```python
from build123d import *

# Parameters (mm, degrees)
SKETCH_1_W           = 10
SKETCH_1_H           = 10
EXTRUDE_2_DEPTH      = 10
EXTRUDE_2_2_DEPTH    = 10
EXTRUDE_2_3_DEPTH    = 10
EXTRUDE_2_4_DEPTH    = 10
SKETCH_2_W           = 100
SKETCH_2_H           = 50
EXTRUDE_3_DEPTH      = 5
SKETCH_4_W           = 100
SKETCH_4_H           = 5
EXTRUDE_4_DEPTH      = 50
SKETCH_7_R           = 4
CUT_EXTRUDE_7_DEPTH  = 100
SKETCH_8_W           = 84
SKETCH_8_H           = 34
CUT_EXTRUDE_9_DEPTH  = 5
CUT_EXTRUDE_12_REACH = 78.195
SKETCH_10_W          = 7
SKETCH_10_H          = 2
CUT_EXTRUDE_13_REACH = 78.195
SKETCH_12_W          = 7
SKETCH_12_H          = 2


with BuildPart() as part:
    # Sketch 1 → Extrude 2 (new body)
    with BuildSketch(Plane(origin=(0, 0, 0), x_dir=(1, 0, 0), z_dir=(0, 1, 0))):
        with Locations((-31.40167364, 31.889818689)):
            Rectangle(SKETCH_1_W, SKETCH_1_H)
    extrude(amount=EXTRUDE_2_DEPTH)



with BuildPart() as body_2:
    # Sketch 1 → Extrude 2 2 (new body)
    with BuildSketch(Plane(origin=(0, 0, 0), x_dir=(1, 0, 0), z_dir=(0, 1, 0))):
        with Locations((-31.40167364, -8.110181311)):
            Rectangle(SKETCH_1_W, SKETCH_1_H)
    extrude(amount=EXTRUDE_2_2_DEPTH)


with BuildPart() as body_3:
    # Sketch 1 → Extrude 2 3 (new body)
    with BuildSketch(Plane(origin=(0, 0, 0), x_dir=(1, 0, 0), z_dir=(0, 1, 0))):
        with Locations((58.59832636, 31.889818689)):
            Rectangle(SKETCH_1_W, SKETCH_1_H)
    extrude(amount=EXTRUDE_2_3_DEPTH)


with BuildPart() as body_4:
    # Sketch 1 → Extrude 2 4 (new body)
    with BuildSketch(Plane(origin=(0, 0, 0), x_dir=(1, 0, 0), z_dir=(0, 1, 0))):
        with Locations((58.59832636, -8.110181311)):
            Rectangle(SKETCH_1_W, SKETCH_1_H)
    extrude(amount=EXTRUDE_2_4_DEPTH)


with BuildPart() as part_1:
    add(part.part)

    add(body_2.part)  # Extrude 3 merges body 2

    add(body_3.part)  # Extrude 3 merges body 3

    add(body_4.part)  # Extrude 3 merges body 4
    # Sketch 2 → Extrude 3 (add)
    with BuildSketch(Plane(origin=(0, 0, 0), x_dir=(1, 0, 0), z_dir=(0, 1, 0))):
        with Locations((13.59832636, 11.889818689)):
            Rectangle(SKETCH_2_W, SKETCH_2_H)
    extrude(amount=-EXTRUDE_3_DEPTH)

    # Sketch 4 → Extrude 4 (add)
    with BuildSketch(Plane.XY.offset(13.110181311)):
        with Locations((13.59832636, 12.5)):
            Rectangle(SKETCH_4_W, SKETCH_4_H)
    extrude(amount=-EXTRUDE_4_DEPTH)

    # Sketch 7 → Cut-Extrude 7 (cut)
    with BuildSketch(Plane.XY.offset(13.110181311)):
        with Locations((-31.20937541, 5)):
            Circle(SKETCH_7_R)
        with Locations((58.59832636, 5)):
            Circle(SKETCH_7_R)
    extrude(amount=-CUT_EXTRUDE_7_DEPTH, mode=Mode.SUBTRACT)

    # Sketch 8 → Cut-Extrude 9 (cut)
    with BuildSketch(Plane(origin=(0, 15, 0), x_dir=(1, 0, 0), z_dir=(0, 1, 0))):
        with Locations((13.59832636, 11.889818689)):
            Rectangle(SKETCH_8_W, SKETCH_8_H)
    extrude(amount=-CUT_EXTRUDE_9_DEPTH, mode=Mode.SUBTRACT)

    # Sketch 10 → Cut-Extrude 12 (cut, up to next)
    with BuildSketch(Plane(origin=(0, 15, 0), x_dir=(1, 0, 0), z_dir=(0, 1, 0)), mode=Mode.PRIVATE) as cut_extrude_12_sk1:
        with Locations((-32.098969847, 27.889818689)):
            Rectangle(SKETCH_10_W, SKETCH_10_H)
    cut_extrude_12_tool1 = extrude(cut_extrude_12_sk1.sketch, amount=-CUT_EXTRUDE_12_REACH, mode=Mode.PRIVATE) & part_1.part
    add(cut_extrude_12_tool1.solids().sort_by_distance((-32.09897, 15, -27.889819))[0], mode=Mode.SUBTRACT)

    # Sketch 12 → Cut-Extrude 13 (cut, up to next)
    with BuildSketch(Plane(origin=(0, 15, 0), x_dir=(1, 0, 0), z_dir=(0, 1, 0)), mode=Mode.PRIVATE) as cut_extrude_13_sk1:
        with Locations((-32.098969847, -4.110181311)):
            Rectangle(SKETCH_12_W, SKETCH_12_H)
    cut_extrude_13_tool1 = extrude(cut_extrude_13_sk1.sketch, amount=-CUT_EXTRUDE_13_REACH, mode=Mode.PRIVATE) & part_1.part
    # Sketch 12 → Cut-Extrude 13 (cut, up to next)
    with BuildSketch(Plane(origin=(0, 15, 0), x_dir=(1, 0, 0), z_dir=(0, 1, 0)), mode=Mode.PRIVATE) as cut_extrude_13_sk2:
        with Locations((59.745274347, 27.889818689)):
            Rectangle(SKETCH_12_W, SKETCH_12_H)
    cut_extrude_13_tool2 = extrude(cut_extrude_13_sk2.sketch, amount=-CUT_EXTRUDE_13_REACH, mode=Mode.PRIVATE) & part_1.part
    # Sketch 12 → Cut-Extrude 13 (cut, up to next)
    with BuildSketch(Plane(origin=(0, 15, 0), x_dir=(1, 0, 0), z_dir=(0, 1, 0)), mode=Mode.PRIVATE) as cut_extrude_13_sk3:
        with Locations((59.745274347, -4.110181311)):
            Rectangle(SKETCH_12_W, SKETCH_12_H)
    cut_extrude_13_tool3 = extrude(cut_extrude_13_sk3.sketch, amount=-CUT_EXTRUDE_13_REACH, mode=Mode.PRIVATE) & part_1.part
    add(cut_extrude_13_tool1.solids().sort_by_distance((-32.09897, 15, 4.110181))[0], mode=Mode.SUBTRACT)
    add(cut_extrude_13_tool2.solids().sort_by_distance((59.745274, 15, -27.889819))[0], mode=Mode.SUBTRACT)
    add(cut_extrude_13_tool3.solids().sort_by_distance((59.745274, 15, 4.110181))[0], mode=Mode.SUBTRACT)


solid = part_1.part
```
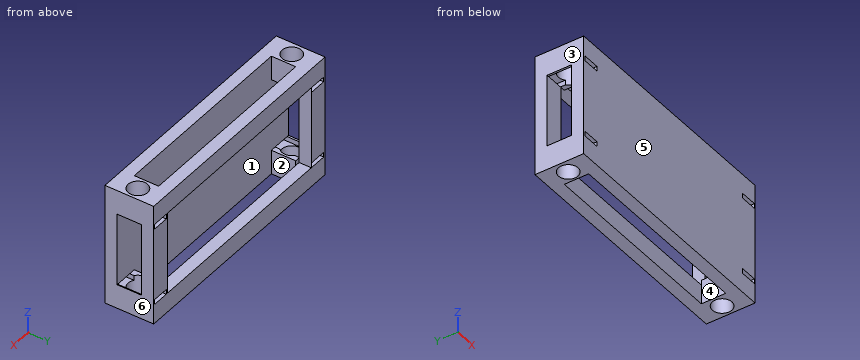
Work out the finished part from the listing and answer in its coordinate system (mm). Face numbers are marked on the shaded views. A direction names the side the tool comes from. Coordinates: 2 decimals unless noted, no trailing zeros. Write each loop counter-clockwise with the first axis right and the second up, starting at its lowest first coordinate (ties: lowest second). Pieces come first, ordered by that corner, then holes. Notation, with made-up numbers: (26, 40.5) - (59, 40.5) arc R9 ccw to (59, 52.5) - close; hole circle Ø8 at (30.25, 87.5). An arc over 180 degrees is marked (long way). Answer as a JSON object with one key per item and string values.
Q1. Consider L1, parallel to X at y = 5, z = 6.5; L2, parallel to Z at x = -29, y = -3; L3, parallel to Y at x = 7, z = -31. Determine where each line is inside the solid, lowest interval first. Write a range as from..to.
Results list:
{"L1": "x = -36.4..-35.21, -27.21..-26.4, 53.6..54.6, 62.6..63.6", "L2": "z = -36.89..-28.89, -26.89..3.11, 5.11..13.11", "L3": "y = -5..0, 10..15"}
Q2. For a pull along X with two mould halves and no side action, classify the marked faces 3, 4, 5 and 6 as pulls with the +X half, pulls with the -X half, needs draft (parallel to the pull), parting line crosses it, or undercut.
Results list:
{"face 3": "pulls with the -X half", "face 4": "undercut", "face 5": "needs draft", "face 6": "pulls with the +X half"}
Q3. Which of the six approach directions +Z, -Z, +X, -X, +Y, -Y give full straight-line access (tool end or side, diameter ignored) to the marked faces 1 and 2?
Results list:
{"face 1": "none", "face 2": "+Z, -Z"}
Q4. Find section C-C (z = -12). Write down the section's boundary in (x, y).
Results list:
{"outline": "(-36.4, -5) - (63.6, -5) - (63.6, 0) - (-36.4, 0) - close; (-36.4, 10) - (-28.4, 10) - (-28.4, 15) - (-36.4, 15) - close; (55.6, 10) - (63.6, 10) - (63.6, 15) - (55.6, 15) - close"}
Q5. Find section D-D (y = 5). State how many separate pieces and enclosed holes the cut face has, plus the area to 3 significant figures.
Results list:
{"separate pieces": "8", "enclosed holes": "0", "area": "75.9 mm^2"}
Q6. Given pin 1 Ø3.5 at (x, y) = (59.5, 3) entering from -Z, flat-ended and moving along its own axis, determine where the tip first touches the part or whether it passes through.
Results list:
{"pin 1": "passes through"}
Q7. Find section B-B (x = 52). Write down the section's boundary in (y, z).
Results list:
{"outline": "(-5, -36.89) - (0, -36.89) - (0, 13.11) - (-5, 13.11) - close; (10, -36.89) - (15, -36.89) - (15, -28.89) - (10, -28.89) - close; (10, 5.11) - (15, 5.11) - (15, 13.11) - (10, 13.11) - close"}
Q8. Find section A-A (z = -32.5). Write down the section's boundary in (x, y).
Results list:
{"outline": "(-36.4, -5) - (63.6, -5) - (63.6, 15) - (-36.4, 15) - close; hole circle Ø8 at (-31.21, 5); hole (-26.4, 0) - (53.6, 0) - (53.6, 10) - (-26.4, 10) - close; hole circle Ø8 at (58.6, 5)"}
